Can you work these out from the model? Positions are in its coordinate system, mm. Face numbers are marked on the shaded views. Give positions to 0.01 mm unless a question says otherwise; leave off trailing zeros. Loops run counter-clockwise (first coordinate to the right, second up) from the corner with the lowest first, then second, coordinate; pieces in that order, holes last.
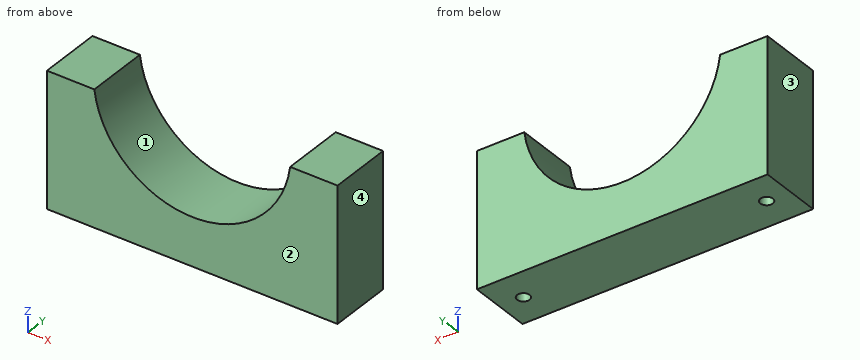
from build123d import *

# Parameters (mm, degrees)
BOSS_EXTRUDE1_DEPTH = 10.16
CUT_EXTRUDE1_DEPTH  = 4.064


with BuildPart() as part:
    # Sketch2 → Boss-Extrude1 (new body)
    with BuildSketch(Plane(origin=(0, 0, 0), x_dir=(1, 0, 0), z_dir=(0, 1, 0))):
        with BuildLine():
            Line((-14.986, -8.89), (-7.366, -8.89))
            ThreePointArc((-7.366, -8.89), (8.382, 4.980973803), (24.13, -8.89))
            Line((24.13, -8.89), (31.75, -8.89))
            Line((31.75, -8.89), (31.75, 12.7))
            Line((31.75, 12.7), (-14.986, 12.7))
            Line((-14.986, 12.7), (-14.986, -8.89))
        make_face()
    extrude(amount=-BOSS_EXTRUDE1_DEPTH)

    # Sketch6 → Cut-Extrude1 (cut)
    with BuildSketch(Plane(origin=(0, 0, -12.7), x_dir=(-1, 0, 0), z_dir=(0, 0, -1))):
        with BuildLine():
            ThreePointArc((-28.9433, -5.08), (-27.94, -6.0833), (-26.9367, -5.08))
            Line((-26.9367, -5.08), (-27.94, -5.08))
            Line((-27.94, -5.08), (-28.9433, -5.08))
        make_face()
        with BuildLine():
            Line((-27.94, -5.08), (-26.9367, -5.08))
            ThreePointArc((-26.9367, -5.08), (-27.94, -4.0767), (-28.9433, -5.08))
            Line((-28.9433, -5.08), (-27.94, -5.08))
        make_face()
        with BuildLine():
            Line((10.1727, -5.08), (11.176, -5.08))
            Line((11.176, -5.08), (12.1793, -5.08))
            ThreePointArc((12.1793, -5.08), (11.176, -4.0767), (10.1727, -5.08))
        make_face()
        with BuildLine():
            Line((12.1793, -5.08), (11.176, -5.08))
            Line((11.176, -5.08), (10.1727, -5.08))
            ThreePointArc((10.1727, -5.08), (11.176, -6.0833), (12.1793, -5.08))
        make_face()
    extrude(amount=-CUT_EXTRUDE1_DEPTH, mode=Mode.SUBTRACT)


solid = part.part
(1) Suppose I cut it at A-A on y = -5.08. List the corners of the cut face in (x, z) for me (3 decimals).
Returned:
outline: (-14.986, -12.7) - (-12.179, -12.7) - (-12.179, -8.636) - (-10.173, -8.636) - (-10.173, -12.7) - (26.937, -12.7) - (26.937, -8.636) - (28.943, -8.636) - (28.943, -12.7) - (31.75, -12.7) - (31.75, 8.89) - (24.13, 8.89) arc R15.875 cw to (-7.366, 8.89) - (-14.986, 8.89) - close
(2) Please list where these lines run through material, in increasing order: probe 1 along X at (y, z) = (-5.08, -9.8); probe 2 along Y at (x, z) = (27.94, -9.7); probe 3 along X at (y, z) = (-8.5, -0.75).
Returned:
probe 1: x = -14.99 to -12.18, -10.17 to 26.94, 28.94 to 31.75
probe 2: y = -10.16 to -6.08, -4.08 to 0
probe 3: x = -14.99 to -2.41, 19.17 to 31.75
(3) Suppose I cut it at C-C on z = 2.5. List the corners of the cut face in (x, y) for me.
Returned:
outline: (-14.99, -10.16) - (-5.09, -10.16) - (-5.09, 0) - (-14.99, 0) - close; (21.86, -10.16) - (31.75, -10.16) - (31.75, 0) - (21.86, 0) - close
(4) Will these pins go through, and if not, where does the flat tip stop? P1, Ø1.5, axis at x = -0.5, y = -2.5, coming from the +Z side (3 decimals); P2, Ø1, axis at x = 18, y = -4, coming from the +Z side; P3, Ø2, axis at x = 28.5, y = -5, coming from the -Z side; P4, Ø1.6, axis at x = 27.94, y = -5.08, coming from the -Z side.
Returned:
P1: stops at z = -1.725
P2: stops at z = -1.34
P3: stops at z = -12.7
P4: stops at z = -8.64
(5) Suppose I cut it at B-B on x = 27.94. List the corners of the cut face in (y, z) for me.
Returned:
outline: (-10.16, -12.7) - (-6.08, -12.7) - (-6.08, -8.64) - (-4.08, -8.64) - (-4.08, -12.7) - (0, -12.7) - (0, 8.89) - (-10.16, 8.89) - close
(6) Suppose I cut it at D-D on y = -7.75. List the corners of the cut face in (x, z) for me (3 decimals).
Returned:
outline: (-14.986, -12.7) - (31.75, -12.7) - (31.75, 8.89) - (24.13, 8.89) arc R15.875 cw to (-7.366, 8.89) - (-14.986, 8.89) - close
(7) Thinking about a two-plate mould opening in X: for the marked faces 1, 2, 3 and 4, which applies, pulls with the +X half, pulls with the -X half, needs draft (parallel to the pull), parting line crosses it, or undercut?
Returned:
face 1: undercut
face 2: needs draft
face 3: pulls with the -X half
face 4: pulls with the +X half
